```python
from build123d import *

# Parameters (mm, degrees)
F0_W     = 1029.208
F0_H     = 311.4294
F1_DEPTH = 120.65
F2_T     = -0.762
F3_W     = 25.4
F3_H     = 52.578
F4_DEPTH = 1029.209
F6_D     = 5.2197
F6_DEPTH = 1.016
F6_TIP   = 1.5681560866
F8_D     = 5.2197
F10_D    = 5.2197


# Not quite as in the source:
# - a feature names something its author has since deleted; it is built from what else it names


with BuildPart() as f1:
    # F0 (on Top) → F1 (new body)
    with BuildSketch(Plane.XY):
        Rectangle(F0_W, F0_H)
    extrude(amount=F1_DEPTH)

    # F2
    f2_openings = [f1.faces().sort_by_distance(p)[0] for p in [
        (0, 0, 0),
    ]]
    offset(amount=F2_T, openings=f2_openings)

    # F3 (on face) → F4 (cut, through all)
    with BuildSketch(Plane(origin=(-514.604, 0, 0), x_dir=(0, -1, 0), z_dir=(-1, 0, 0))):
        with Locations((143.0147, 26.289)):
            Rectangle(F3_W, F3_H)
    extrude(amount=-F4_DEPTH, mode=Mode.SUBTRACT)

    # F6
    with Locations(Plane(origin=(0, 155.7147, 0), x_dir=(-1, 0, 0), z_dir=(0, 1, 0))):
        with Locations((-488.95, 7.366), (488.95, 7.366), (0, 7.366), (-244.475, 7.366), (244.475, 7.366)):
            Hole(F6_D / 2, depth=F6_DEPTH)
            with Locations((0, 0, -(F6_DEPTH + F6_TIP / 2))):  # 118° drill point
                Cone(0, F6_D / 2, F6_TIP, mode=Mode.SUBTRACT)

    # F8 (through all)
    with Locations(Plane(origin=(-514.604, 0, 0), x_dir=(0, -1, 0), z_dir=(-1, 0, 0))):
        with Locations((-116.0907, 7.366), (-1.7907, 7.366), (112.5093, 7.366)):
            Hole(F8_D / 2)

    # F10 (through all)
    with Locations(Plane(origin=(-514.604, 0, 0), x_dir=(0, -1, 0), z_dir=(-1, 0, 0))):
        with Locations((-127, 76.2), (0, 76.2), (127, 76.2)):
            Hole(F10_D / 2)


solid = f1.part
```
Can you work these out from the model? Positions are in its coordinate system, mm. A direction names the side the tool comes from. Round coordinates to 2 decimals unless told otherwise and drop trailing zeros. Loops run counter-clockwise (first coordinate to the right, second up) from the corner with the lowest first, then second, coordinate; pieces in that order, holes last. Notation, with made-up numbers: (43.5, 1) -> (75.5, 1) arc R23 ccw to (75.5, 36) -> close; hole circle Ø2 at (85, 69.5). An arc over 180 degrees is marked (long way). One line per item, written item: value. Start each with the question number.
1. If we section it at C-C, the plane y = -37: Write out the boundary of the cut face in (x, z), then the cut area to 3 significant figures.
2. If we mould it in two halves opening along Y, with no side actions, what happens to faces 1 (the flat face through (513.842, -2, 59)), 2 (the flat face through (-2.4, -155.2, 52.578)), 3 (the flat face through (-7, 155.715, 59))? For each: pulls with the +Y half, pulls with the -Y half, needs draft (parallel to the pull), parting line crosses it, or undercut.
3. If we section it at A-A, the plane z = 92.5: Write out the boundary of the cut face in (x, y), then the cut area to 3 significant figures.
4. If I drill on probe 1 along Y at (x, z) = (57.5, 54); probe 2 along X at (y, z) = (86, 111.5); probe 3 along Z at (x, y) = (-514, -127), over which ranges is the centre line in solid material (lowest first)?
5. For faces 4 (the flat face through (-514.604, -2, 59)), 5 (the flat face through (-513.842, -2, 59)), which set-ups out of +Z, -Z, +X, -X, +Y, -Y let a thin tool reach every point of the face, with its end or its side?
6. If we section it at B-B, the plane x = -310.5: Write out the boundary of the cut face in (y, z).
7. For pin 1 (4.5 mm diameter, centred on x = 244.475, z = 7.366, fed in from +Y); pin 2 (5 mm diameter, centred on x = -226.5, y = -42.5, fed in from -Z); pin 3 (7 mm diameter, centred on x = 0, z = 7.366, fed in from -Y), each with a flat end and sliding along its axis, tell me the tip position at first contact or that it passes through.
Calculated:
1. outline: (-514.6, 0) -> (-513.84, 0) -> (-513.84, 119.89) -> (513.84, 119.89) -> (513.84, 0) -> (514.6, 0) -> (514.6, 120.65) -> (-514.6, 120.65) -> close
1. area: 967 mm²
2. face 1: undercut
2. face 2: needs draft
2. face 3: pulls with the +Y half
3. outline: (-514.6, -155.71) -> (514.6, -155.71) -> (514.6, 155.71) -> (-514.6, 155.71) -> close; hole (-513.84, -154.95) -> (513.84, -154.95) -> (513.84, 154.95) -> (-513.84, 154.95) -> close
3. area: 2,040 mm²
4. probe 1: y = -155.71 to -154.95, 154.95 to 155.71
4. probe 2: x = -514.6 to -513.84, 513.84 to 514.6
4. probe 3: z = 0 to 73.59, 78.81 to 120.65
5. face 4: +Z, -Z, -X, +Y, -Y
5. face 5: -Z
6. outline: (-155.71, 52.58) -> (-154.95, 52.58) -> (-154.95, 119.89) -> (154.95, 119.89) -> (154.95, 0) -> (155.71, 0) -> (155.71, 120.65) -> (-155.71, 120.65) -> close
7. pin 1: passes through
7. pin 2: stops at z = 119.89
7. pin 3: stops at y = 154.95
